Geometry: see drawing. Coordinates: mm, zero at the bounding-box minimum. Round coordinates to 2 decimals unless told otherwise and drop trailing zeros. Write each loop counter-clockwise with the first axis right and the second up, starting at its lowest first coordinate (ties: lowest second). Pieces come first, ordered by that corner, then holes.
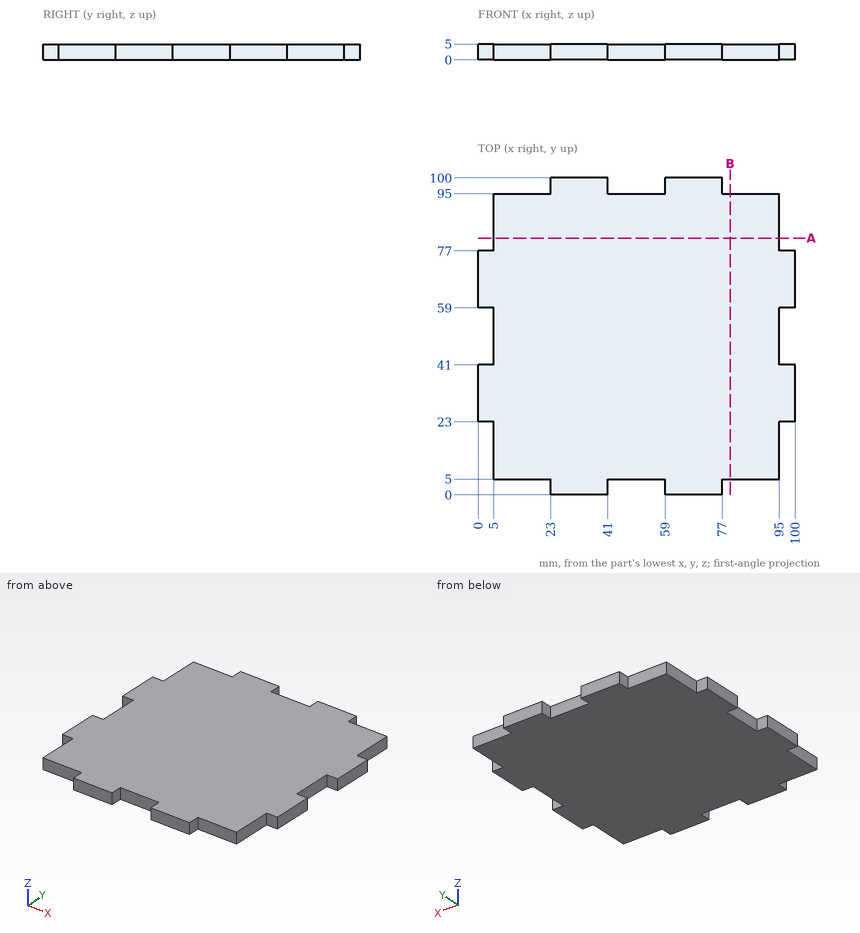
Q1. Line query: line 1 (X direction, y = 19.5, z = 3.65). Output: solid intervals per line, ascending.
Q2. Section query A-A, the plane y = 81. Output: boundary loops of the cut face in (x, z).
Q3. Pin query (flat end, axial travel): P1, Ø12, axis at x = 24.5, y = 89.5, coming from the -Z side; P2, Ø1.5, axis at y = 2.5, z = 1.5, coming from the -X side; P3, Ø1.5, axis at x = 2.5, z = 2.5, coming from the +Y side; P4, Ø1.5, axis at x = 90.5, z = 2.5, coming from the -Y side. Return the tip coordinate at first contact, or that it passes through.
Filled in:
1. line 1: x = 5 to 95
2. outline: (5, 0) - (95, 0) - (95, 5) - (5, 5) - close
3. P1: stops at z = 0
3. P2: stops at x = 23
3. P3: stops at y = 77
3. P4: stops at y = 5
